Geometry check sheet. Reference: the model listing, model coordinates, mm. Face numbers are marked on the shaded views. Coordinates: 2 decimals unless noted, no trailing zeros. Loops run counter-clockwise (first coordinate to the right, second up) from the corner with the lowest first, then second, coordinate; pieces in that order, holes last. Notation, with made-up numbers: (21.25, 75) - (52.25, 75) arc R17 cw to (52.25, 96) - close; hole circle Ø1 at (-24.5, -38.75). An arc over 180 degrees is marked (long way). One line per item, written item: value.
from build123d import *

# Parameters (mm, degrees)
BOSS_EXTRUDE1_DEPTH = 4
SKETCH3_W           = 24.197009966
SKETCH3_H           = 2
CUT_EXTRUDE1_DEPTH  = 51
SKETCH5_W           = 4
SKETCH5_H           = 50
BOSS_EXTRUDE2_DEPTH = 20
CUT_EXTRUDE2_DEPTH  = 17.78
SKETCH7_R           = 1.5875
CUT_EXTRUDE3_DEPTH  = 5
SKETCH8_W           = 1.605980069
SKETCH8_H           = 2.54
BOSS_EXTRUDE3_DEPTH = 4.064


with BuildPart() as part:
    # Sketch2 → Boss-Extrude1 (new body)
    with BuildSketch(Plane.XY):
        Polygon((50, 42.164), (50, 50), (1.605980069, 50), (1.605980069, 47.46), (0, 47.46), (0, 0), (50, 0), (50, 7.874), (39.535978332, 11.684), (39.535978332, 38.354), align=None)
    extrude(amount=BOSS_EXTRUDE1_DEPTH)

    # Sketch3 → Cut-Extrude1 (cut, through all)
    with BuildSketch(Plane(origin=(0, 50, 0), x_dir=(1, 0, 0), z_dir=(0, 1, 0))):
        with Locations((37.901495017, -1)):
            Rectangle(SKETCH3_W, SKETCH3_H)
    extrude(amount=-CUT_EXTRUDE1_DEPTH, mode=Mode.SUBTRACT)

    # Sketch5 → Boss-Extrude2 (add)
    with BuildSketch(Plane.ZY):
        with Locations((2, 25)):
            Rectangle(SKETCH5_W, SKETCH5_H)
    extrude(amount=BOSS_EXTRUDE2_DEPTH)

    # Sketch6 → Cut-Extrude2 (cut)
    with BuildSketch(Plane.ZY.offset(20)):
        with BuildLine():
            Line((3.5, 19.656649926), (3.5, 30.343350074))
            ThreePointArc((3.5, 30.343350074), (3.751975341, 30.266115496), (4, 30.177005892))
            Line((4, 30.177005892), (4, 19.822994108))
            ThreePointArc((4, 19.822994108), (3.751975341, 19.733884504), (3.5, 19.656649926))
        make_face()
        with BuildLine():
            Line((0.5, 19.656649926), (0.5, 30.343350074))
            ThreePointArc((0.5, 30.343350074), (0.248024659, 30.266115496), (0, 30.177005892))
            Line((0, 30.177005892), (0, 19.822994108))
            ThreePointArc((0, 19.822994108), (0.248024659, 19.733884504), (0.5, 19.656649926))
        make_face()
    extrude(amount=-CUT_EXTRUDE2_DEPTH, mode=Mode.SUBTRACT)

    # Sketch7 → Cut-Extrude3 (cut, through all)
    with BuildSketch(Plane(origin=(0, 0, 0), x_dir=(-1, 0, 0), z_dir=(0, 0, -1))):
        with Locations((6.284, 25)):
            Circle(SKETCH7_R)
    extrude(amount=-CUT_EXTRUDE3_DEPTH, mode=Mode.SUBTRACT)

    # Sketch8 → Boss-Extrude3 (add)
    with BuildSketch(Plane.XY.offset(4)):
        with Locations((0.802990035, 48.73)):
            Rectangle(SKETCH8_W, SKETCH8_H)
    extrude(amount=-BOSS_EXTRUDE3_DEPTH)


solid = part.part
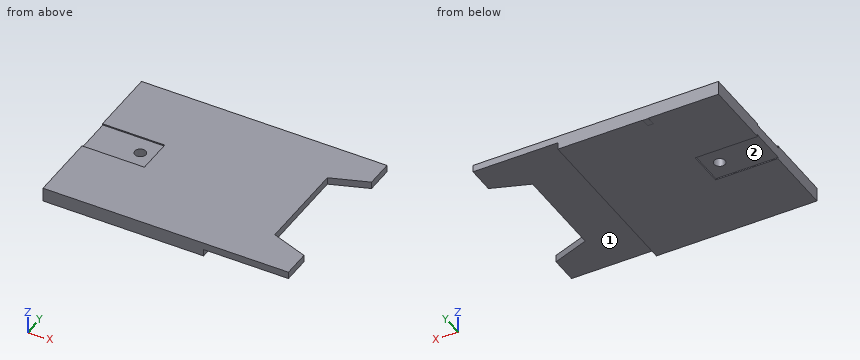
(1) Cross-section at B-B on z = 1.3. Record the cut outline in (x, y) (1 decimal), and give its area (3 significant figures).
Reply:
outline: (-20, 0) - (25.8, 0) - (25.8, 50) - (-20, 50) - close; hole circle Ø3.2 at (-6.3, 25)
area: 2,280 mm2
(2) Material ranges on probe 1 along X at (y, z) = (35.5, 1); probe 2 along Z at (x, y) = (-14, 16); probe 3 along Y at (x, z) = (-6, 3.15), recorded low to high. Write a range as from..to.
Reply:
probe 1: -20..25.8
probe 2: 0..4
probe 3: 0..23.44, 26.56..50
(3) Release check for a two-part mould opening along Y. For the marked faces 1 and 2 record: pulls with the +Y half, pulls with the -Y half, needs draft (parallel to the pull), parting line crosses it, or undercut.
Reply:
face 1: needs draft
face 2: undercut
(4) Cross-section at D-D on x = -3.5. Record the cut outline in (y, z), and give its area (3 significant figures).
Reply:
outline: (0, 0) - (19.82, 0) arc R5.55 cw to (19.66, 0.5) - (30.34, 0.5) arc R5.55 cw to (30.18, 0) - (50, 0) - (50, 4) - (30.18, 4) arc R5.55 cw to (30.34, 3.5) - (19.66, 3.5) arc R5.55 cw to (19.82, 4) - (0, 4) - close
area: 189 mm2
(5) Go/stop test with flat-tipped pins: pin 1 Ø3 at (x, y) = (5, 32) entering from -Z; pin 2 Ø4 at (x, y) = (-6.284, 25) entering from -Z; pin 3 Ø1.6 at (y, z) = (19, 0.5) entering from +X. Record where each tip stops, or that it passes through.
Reply:
pin 1: z = 0
pin 2: z = 0.5
pin 3: x = 25.8
(6) Cross-section at C-C on y = 13. Record the cut outline in (x, z), and give its area (3 significant figures).
Reply:
outline: (-20, 0) - (25.8, 0) - (25.8, 2) - (39.54, 2) - (39.54, 4) - (-20, 4) - close
area: 211 mm2
(7) Cross-section at A-A on y = 25. Record the cut outline in (x, z), and give its area (3 significant figures).
Reply:
outline: (-20, 0.5) - (-7.87, 0.5) - (-7.87, 3.5) - (-20, 3.5) - close; (-4.7, 0.5) - (-2.22, 0.5) - (-2.22, 0) - (25.8, 0) - (25.8, 2) - (39.54, 2) - (39.54, 4) - (-2.22, 4) - (-2.22, 3.5) - (-4.7, 3.5) - close
area: 183 mm2
